Study the drawing (mm; zero at the part's minimum x, y, z) and answer. A direction names the side the tool comes from. Coordinates: 2 decimals unless noted, no trailing zeros. Write each loop counter-clockwise with the first axis right and the second up, starting at its lowest first coordinate (ties: lowest second). Pieces come first, ordered by that corner, then holes. Notation, with made-up numbers: (-30.5, -17) -> (-26.5, -17) arc R24 cw to (-26.5, -5) -> close; hole circle Ø8 at (-17.75, 51.5). An arc over 180 degrees is marked (long way). Write each question's results on one line, items separated by ' | '. Start each with the question number.
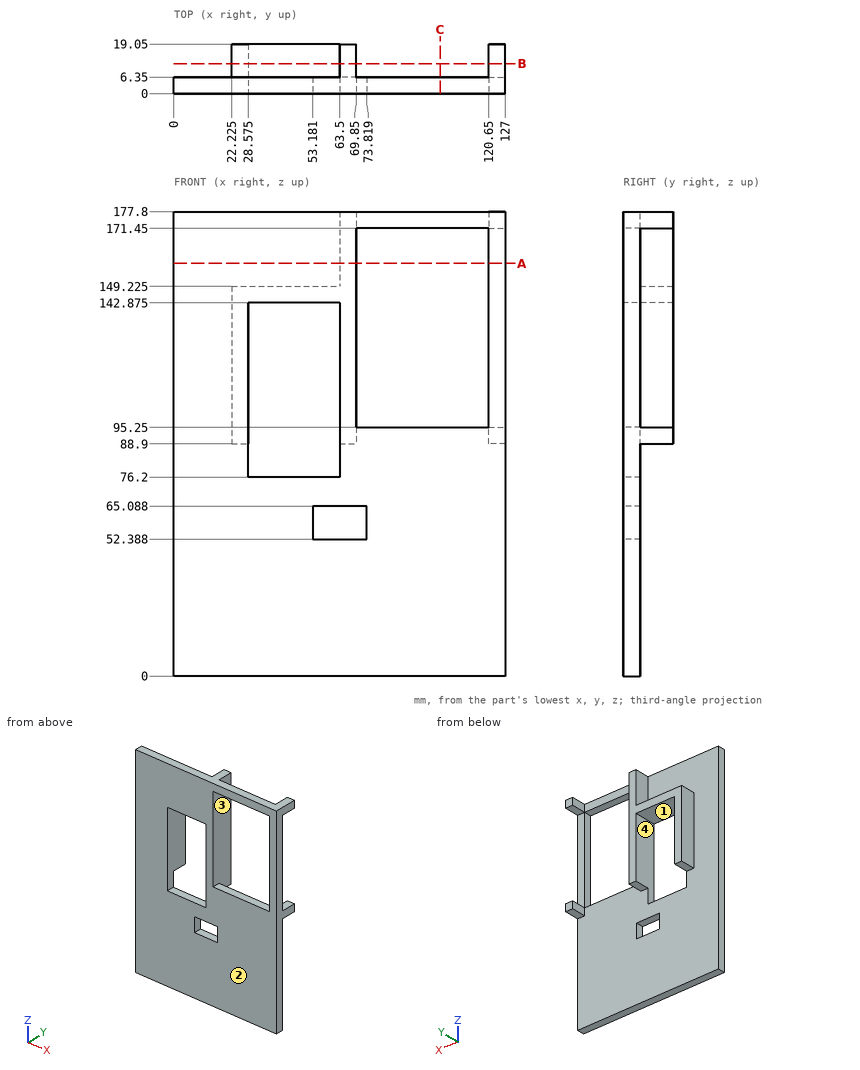
1. Find the intervals of material crossed by L1, parallel to Z at x = 82, y = 2.25; L2, parallel to Z at x = 50.5, y = 4.75 (1 decimal); L3, parallel to Y at x = 45.5, z = 64, in increasing order.
2. For the marked faces 3 and 4, determine the directions among +Z, -Z, +X, -X, +Y, -Y from which every point of the face is accessible in a straight line to the end or side of a thin tool.
3. Find section A-A on z = 158. Give the vertices of the cut face in (x, y).
4. Determine the mould class of the marked faces 1 and 2 for opening direction X: pulls with the +X half, pulls with the -X half, needs draft (parallel to the pull), parting line crosses it, or undercut.
5. Find section C-C on x = 102. Give the vertices of the cut face in (y, z), and give its area (3 significant figures).
6. Given pin 1 Ø10 at (x, y) = (53, 14) entering from +Z (1 decimal); pin 2 Ø1.9 at (x, y) = (65.5, 12) entering from -Z; pin 3 Ø8 at (x, z) = (48, 37) entering from +Y, each flat-ended and moving along its own axis, determine where each tip first touches the part or whether it passes through.
7. Find section B-B on y = 11.5. Give the number of separate pieces and of enclosed holes in the cut face, and give its area (3 significant figures).
Ans:
1) L1: z = 0 to 95.25, 171.45 to 177.8 | L2: z = 0 to 76.2, 142.9 to 177.8 | L3: y = 0 to 6.35
2) face 3: +Y | face 4: +Y, -Y
3) outline: (0, 0) -> (69.85, 0) -> (69.85, 19.05) -> (63.5, 19.05) -> (63.5, 6.35) -> (0, 6.35) -> close; (120.65, 0) -> (127, 0) -> (127, 6.35) -> (120.65, 6.35) -> close
4) face 1: undercut | face 2: needs draft
5) outline: (0, 0) -> (6.35, 0) -> (6.35, 95.25) -> (0, 95.25) -> close; (0, 171.45) -> (6.35, 171.45) -> (6.35, 177.8) -> (0, 177.8) -> close | area: 645 mm²
6) pin 1: stops at z = 149.2 | pin 2: stops at z = 88.9 | pin 3: stops at y = 6.35
7) separate pieces: 3 | enclosed holes: 0 | area: 1,250 mm²
